Check sheet for the modelled part. Datum: model origin and axes. Units: mm. Face numbers are marked on the shaded views. A direction names the side the tool comes from. Round coordinates to 2 decimals unless told otherwise and drop trailing zeros. Order: outer loops, then holes, each group sorted by start corner. A loop starts at its lowest first (then second) coordinate and runs counter-clockwise, first axis right, second up. Notation, with made-up numbers: M 76.25,-37 L 99.25,-37 A14 ccw 99.25,-24 Z; hole C 13.25,37 d9. An arc over 180 degrees is marked long. One line per item, written item: value. Start each with the question number.
(1) Access from +Z, -Z, +X, -X, +Y, -Y to the whole of each face (thin tool, end or side, straight path). Record for the marked faces 1, 2, 3 and 4.
(2) Depth check by flat-ended pin: pin 1 Ø8 at (x, z) = (10, 43.5) entering from +Y; pin 2 Ø5 at (x, y) = (15.78, 98.05) entering from +Z; pin 3 Ø4 at (y, z) = (45, -8.5) entering from -X; pin 4 Ø10 at (y, z) = (9, 33) entering from -X. Enter the tip coordinate at first touch or a pass-through.
(3) Cross-section at A-A, the plane x = 12.7. Count the separate pieces of the cut face and the enclosed holes in it, and give its area (3 significant figures).
(4) Thickness scan on L1, parallel to Y at x = 12, z = -2 (3 decimals); L2, parallel to Y at x = 15, z = -5 (3 decimals); L3, parallel to Z at x = 17.5, y = 85. Record the ranges inside material, lowest first.
(5) Cross-section at B-B, the plane y = 28.5. Enter the section's corners in (x, z), and give its area (3 significant figures).
(6) Cross-section at C-C, the plane z = 28.5. Enter the section's corners in (x, y) (3 decimals), and give its area (3 significant figures).
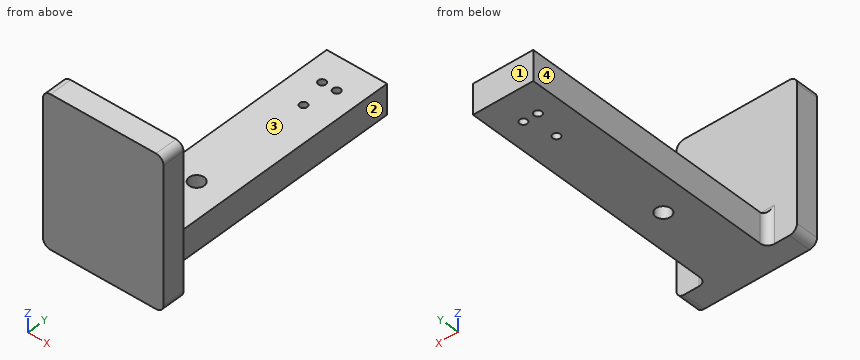
Autodesk Inventor part; units mm, degrees
ref_plane "YZ Plane" through (0, 0, 0) normal (1, 0, 0) x (0, 1, 0)
ref_plane "XZ Plane" through (0, 0, 0) normal (0, 1, 0) x (-1, 0, 0)
ref_plane "XY Plane" through (0, 0, 0) normal (0, 0, 1) x (1, 0, 0)
sketch "Sketch1" plane through (0, 0, 0) normal (1, 0, 0) x (0, 1, 0)
  line L0 (0, 0) -> (111.125, 0)
  line L1 (111.125, 0) -> (111.125, -12.7)
  line L2 (111.125, -12.7) -> (-9.525, -12.7)
  line L3 (-9.525, -12.7) -> (-9.525, 50.8)
  line L4 (-9.525, 50.8) -> (0, 50.8)
  line L5 (0, 50.8) -> (0, 0)
  line L6 (0, 0) -> (0, -12.7)
  dimension "d0" = 111.125
  dimension "d1" = 12.7
  dimension "d2" = 120.65
  dimension "d3" = 63.5
extrude "Extrusion1" add sketch "Sketch1" along normal blind 25.4 contours L0 L1 L2 L6
sketch "Sketch2" plane through (0, 0, 0) normal (0, 0, 1) x (1, 0, 0)
  line L0 (0, 0) -> (25.4, 0)
  circle A0 centre (12.7, 34.925) radius 3.175
  circle A1 centre (12.7, 85.725) radius 1.5875
  circle A2 centre (15.78, 98.0459) radius 1.5875
  line L1 (25.4, 111.125) -> (25.4, 0)
  line L2 (0, 111.125) -> (0, 0)
  circle A3 centre (9.62, 98.0459) radius 1.5875
  line L3 (0, 111.125) -> (25.4, 111.125)
  line L4 (12.7, 111.125) -> (12.7, 0)
  dimension "d7" = 6.35
  dimension "d8" = 3.175
  dimension "d9" = 34.925
  dimension "d10" = 50.8
  dimension "d11" = 3.175
  dimension "d12" = 12.7
  dimension "d17" = 3.175
  dimension "d18" = 12.7
  dimension "d22" = 3.08
  dimension "d23" = 3.08
extrude "Extrusion2" cut sketch "Sketch2" against normal blind 25.4 contours L4 A0 | A0 L4 | L4 A1 | A1 L4 | A2 | A3
extrude "Extrusion3" add sketch "Sketch1" along normal blind 38.1 and the other way blind 12.7 contours L6 L2 L3 L4 L5
fillet "Fillet1" radius 3.175 3 edges at (25.4, 0, -6.35) (12.7, 0, 0) (0, 0, -6.35)
fillet "Fillet2" radius 3.175 4 edges at (38.1, -4.7625, -12.7) (38.1, -4.7625, 50.8) (-12.7, -4.7625, 50.8) (-12.7, -4.7625, -12.7)
properties part number "Based"
Values found:
1. face 1: +Z, -Z, +X, -X, +Y
1. face 2: +Z, -Z, +X, +Y
1. face 3: +Z, +X, -X, +Y
1. face 4: +Z, -Z, -X, +Y
2. pin 1: y = 0
2. pin 2: z = 0
2. pin 3: x = 0
2. pin 4: through
3. separate pieces: 3
3. enclosed holes: 0
3. area: 1,900 mm^2
4. L1: -9.525 to 31.828, 38.022 to 84.3, 87.15 to 111.125
4. L2: -9.525 to 32.736, 37.114 to 96.663, 99.429 to 111.125
4. L3: -12.7 to 0
5. outline: M 0,-12.7 L 25.4,-12.7 L 25.4,0 L 0,0 Z
5. area: 323 mm^2
6. outline: M -12.7,-9.525 L 38.1,-9.525 L 38.1,0 L -12.7,0 Z
6. area: 484 mm^2
